Verification items for the finished model (mm, model axes). Coordinates: 2 decimals unless noted, no trailing zeros. Order: outer loops, then holes, each group sorted by start corner. A loop starts at its lowest first (then second) coordinate and runs counter-clockwise, first axis right, second up. Notation, with made-up numbers: M 72,59 L 126,59 A13 ccw 126,72 Z; hole C 30,5.5 d4. An arc over 180 degrees is marked long. Return JSON: item names as keys, results as strings.
```python
from build123d import *

# Parameters (mm, degrees)
SKETCH1_R      = 1
EXTRUDE1_DEPTH = 0.6
FILLET1_R      = 1.2


with BuildPart() as part:
    # Sketch1 → Extrude1 (new body, symmetric)
    with BuildSketch(Plane(origin=(0, 0, 0), x_dir=(0, 0, -1), z_dir=(1, 0, 0))):
        with BuildLine():
            Line((-0.16143476, 9.24859118), (-0.231244385, 13.247981961))
            ThreePointArc((-0.231244385, 13.247981961), (-2.73314864, 12.965045257), (-5.136358645, 12.213939572))
            Line((-5.136358645, 12.213939572), (-5.866544122, 9.285325583))
            ThreePointArc((-5.866544122, 9.285325583), (0, -11.85), (5.866544122, 9.285325583))
            Line((5.866544122, 9.285325583), (5.136358645, 12.213939572))
            ThreePointArc((5.136358645, 12.213939572), (2.73314864, 12.965045257), (0.231244385, 13.247981961))
            Line((0.231244385, 13.247981961), (0.16143476, 9.24859118))
            ThreePointArc((0.16143476, 9.24859118), (0, -9.25), (-0.16143476, 9.24859118))
        make_face()
        with Locations((-2.53014565, 11.207549834)):
            Circle(SKETCH1_R, mode=Mode.SUBTRACT)
        with Locations((2.53014565, 11.207549834)):
            Circle(SKETCH1_R, mode=Mode.SUBTRACT)
    extrude(amount=EXTRUDE1_DEPTH, both=True)

    # Fillet1
    fillet1_edges = [part.edges().sort_by_distance(p)[0] for p in [
        (0, 12.213939572, -5.136358645),
        (0, 9.285325583, -5.866544122),
        (0, 9.285325583, 5.866544122),
        (0, 12.213939572, 5.136358645),
    ]]
    fillet(fillet1_edges, radius=FILLET1_R)


solid = part.part
```
Q1. Cross-section at A-A, the plane y = -8.75. Record the boundary of the cut face in (x, z).
Values:
{"outline": "M -0.6,-7.81 L 0.6,-7.81 L 0.6,-3 L -0.6,-3 Z; M -0.6,3 L 0.6,3 L 0.6,7.81 L -0.6,7.81 Z"}
Q2. Cross-section at D-D, the plane z = 2. Record the boundary of the cut face in (x, y).
Values:
{"outline": "M -0.6,-11.67 L 0.6,-11.67 L 0.6,-9.03 L -0.6,-9.03 Z; M -0.6,9.03 L 0.6,9.03 L 0.6,10.36 L -0.6,10.36 Z; M -0.6,12.06 L 0.6,12.06 L 0.6,13.1 L -0.6,13.1 Z"}
Q3. Draft check along Z on faces 1 (the face through (-0.6, 7.3, 6)), 2 (the face through (0.01, 13.02, -2.45)), 3 (the face through (-0.008, 10.231, -2.313)), 4 (the face through (0.01, -9.24, -0.4)). Enter one of: pulls with the +Z half, pulls with the -Z half, needs draft (parallel to the pull), parting line crosses it, or undercut.
Values:
{"face 1": "needs draft", "face 2": "pulls with the -Z half", "face 3": "undercut", "face 4": "undercut"}
Q4. Material ranges on line 1 along Z through (x, y) = (-0.1, 10.75); line 2 along Y through (x, z) = (-0.15, 1.75); line 3 along Y through (x, z) = (0.4, 3.75), recorded low to high.
Values:
{"line 1": "-5.5 to -3.42, -1.64 to -0.19, 0.19 to 1.64, 3.42 to 5.5", "line 2": "-11.71 to -9.08, 9.08 to 10.58, 11.83 to 13.13", "line 3": "-11.21 to -8.46, 8.46 to 12.71"}
Q5. Cross-section at C-C, the plane x = 0.1. Record the boundary of the cut face in (y, z).
Values:
{"outline": "M 9.04,-6.25 A1.2 cw 9.75,-5.75 L 11.61,-5.29 A1.2 ccw 12.45,-4.53 A13.25 ccw 13.25,-0.23 L 9.25,-0.16 A9.25 cw long 9.25,0.16 L 13.25,0.23 A13.25 ccw 12.45,4.53 A1.2 ccw 11.61,5.29 L 9.75,5.75 A1.2 cw 9.04,6.25 A11.38 ccw long Z; hole C 11.21,-2.53 d2; hole C 11.21,2.53 d2"}
Q6. Cross-section at B-B, the plane z = -8. Record the boundary of the cut face in (x, y).
Values:
{"outline": "M -0.6,-8.56 L 0.6,-8.56 L 0.6,-4.64 L -0.6,-4.64 Z; M -0.6,4.64 L 0.6,4.64 L 0.6,7.63 L -0.6,7.63 Z"}
